Verification items for the finished model (mm, model axes). A direction names the side the tool comes from. Round coordinates to 2 decimals unless told otherwise and drop trailing zeros. Order: outer loops, then holes, each group sorted by start corner. A loop starts at its lowest first (then second) coordinate and runs counter-clockwise, first axis right, second up. Notation, with made-up numbers: (36, 64) -> (87, 64) arc R11 cw to (87, 76) -> close; hole circle Ø9 at (55.5, -25). An arc over 180 degrees is marked (long way). Put each result on its own line as item: value.
```python
from build123d import *

# Parameters (mm, degrees)
BOSS_EXTRUDE1_DEPTH = 15
BOSS_EXTRUDE2_DEPTH = 42
CUT_EXTRUDE1_REACH  = 101.75
SKETCH2_R           = 3.5


with BuildPart() as part:
    # Sketch1 → Boss-Extrude1 (new body)
    with BuildSketch(Plane(origin=(0, 0, 0), x_dir=(1, 0, 0), z_dir=(0, 1, 0))):
        with BuildLine():
            Line((74, 0), (27, 0))
            Line((27, 0), (27, -31))
            Line((27, -31), (62, -31))
            Line((62, -31), (112, -23))
            Line((112, -23), (112, -9))
            Line((112, -9), (83, -9))
            ThreePointArc((83, -9), (76.636038969, -6.363961031), (74, 0))
        make_face()
        with BuildLine():
            Line((27, 31), (27, 0))
            Line((27, 0), (74, 0))
            ThreePointArc((74, 0), (76.636038969, 6.363961031), (83, 9))
            Line((83, 9), (112, 9))
            Line((112, 9), (112, 23))
            Line((112, 23), (62, 31))
            Line((62, 31), (27, 31))
        make_face()
    extrude(amount=BOSS_EXTRUDE1_DEPTH)

    # Sketch1_3 → Boss-Extrude2 (add)
    with BuildSketch(Plane(origin=(0, 0, 0), x_dir=(1, 0, 0), z_dir=(0, 1, 0))):
        Polygon((7, 20), (0, 20), (0, 0), (27, 0), (27, 31), (7, 31), align=None)
        Polygon((27, 0), (0, 0), (0, -20), (7, -20), (7, -31), (27, -31), align=None)
    extrude(amount=BOSS_EXTRUDE2_DEPTH)

    # Sketch2 → Cut-Extrude1 (cut, up to next)
    with BuildSketch(Plane(origin=(27, 0, 0), x_dir=(0, 0, -1), z_dir=(1, 0, 0)), mode=Mode.PRIVATE) as cut_extrude1_sk1:
        with Locations((0, 33)):
            Circle(SKETCH2_R)
    cut_extrude1_tool1 = extrude(cut_extrude1_sk1.sketch, amount=-CUT_EXTRUDE1_REACH, mode=Mode.PRIVATE) & part.part
    # Sketch2 → Cut-Extrude1 (cut, up to next)
    with BuildSketch(Plane(origin=(27, 0, 0), x_dir=(0, 0, -1), z_dir=(1, 0, 0)), mode=Mode.PRIVATE) as cut_extrude1_sk2:
        Polygon((-31, 30), (-8.431282416, 42), (-31, 42), align=None)
    cut_extrude1_tool2 = extrude(cut_extrude1_sk2.sketch, amount=-CUT_EXTRUDE1_REACH, mode=Mode.PRIVATE) & part.part
    # Sketch2 → Cut-Extrude1 (cut, up to next)
    with BuildSketch(Plane(origin=(27, 0, 0), x_dir=(0, 0, -1), z_dir=(1, 0, 0)), mode=Mode.PRIVATE) as cut_extrude1_sk3:
        Polygon((31, 42), (8.431282416, 42), (31, 30), align=None)
    cut_extrude1_tool3 = extrude(cut_extrude1_sk3.sketch, amount=-CUT_EXTRUDE1_REACH, mode=Mode.PRIVATE) & part.part
    add(cut_extrude1_tool1.solids().sort_by_distance((27, 33, 0))[0], mode=Mode.SUBTRACT)
    add(cut_extrude1_tool2.solids().sort_by_distance((27, 38, 23.477094))[0], mode=Mode.SUBTRACT)
    add(cut_extrude1_tool3.solids().sort_by_distance((27, 38, -23.477094))[0], mode=Mode.SUBTRACT)


solid = part.part
```
Item 1: Depth check by flat-ended pin: pin 1 Ø4 at (x, z) = (52, -14) entering from +Y; pin 2 Ø5.5 at (x, y) = (2.5, 12.5) entering from -Z; pin 3 Ø5 at (y, z) = (28, -20.5) entering from +X. Enter the tip coordinate at first touch or a pass-through.
Geometry check:
pin 1: y = 15
pin 2: z = -20
pin 3: x = 27
Item 2: Release check for a two-part mould opening along Z. For faces 6 (the face through (7, 18, -26)), 7 (the face through (97, 7, -9)), 8 (the face through (29, 11, -31)) record: pulls with the +Z half, pulls with the -Z half, needs draft (parallel to the pull), parting line crosses it, or undercut.
Geometry check:
face 6: needs draft
face 7: undercut
face 8: pulls with the -Z half
Item 3: Sectioned sample at C-C, the plane x = 25. Record the boundary of the cut face in (y, z), then the cut area to 3 significant figures.
Geometry check:
outline: (0, -31) -> (30, -31) -> (42, -8.43) -> (42, 8.43) -> (30, 31) -> (0, 31) -> close; hole circle Ø7 at (33, 0)
area: 2,290 mm2
Item 4: Tool access check on faces 1 (the face through (4, 18, -20)), 2 (the face through (87, 7, 27)), 3 (the face through (13.689, 36.084, -19.558)), 4 (the face through (3, 18, 20)), 5 (the face through (59, 15, 0)). Record the directions out of +Z, -Z, +X, -X, +Y, -Y that give a thin tool (end or side, any length) a straight path to the whole face; none if there is none.
Geometry check:
face 1: -Z, -X, +Y, -Y
face 2: +Z, +X, +Y, -Y
face 3: -Z, +X, -X, +Y
face 4: +Z, -X, +Y, -Y
face 5: +Z, -Z, +X, +Y
Item 5: Material ranges on line 1 along Y through (x, z) = (16, 0); line 2 along X through (y, z) = (35.5, -6); line 3 along Y through (x, z) = (53, -3.5), recorded low to high.
Geometry check:
line 1: 0 to 29.5, 36.5 to 42
line 2: 0 to 27
line 3: 0 to 15
Item 6: Sectioned sample at D-D, the plane y = 33. Record the boundary of the cut face in (x, z), then the cut area to 3 significant figures.
Geometry check:
outline: (0, -20) -> (7, -20) -> (7, -25.36) -> (27, -25.36) -> (27, -3.5) -> (0, -3.5) -> close; (0, 3.5) -> (27, 3.5) -> (27, 25.36) -> (7, 25.36) -> (7, 20) -> (0, 20) -> close
area: 1,110 mm2
Item 7: Sectioned sample at A-A, the plane x = 89. Record the boundary of the cut face in (y, z).
Geometry check:
outline: (0, -26.68) -> (15, -26.68) -> (15, -9) -> (0, -9) -> close; (0, 9) -> (15, 9) -> (15, 26.68) -> (0, 26.68) -> close
Item 8: Sectioned sample at B-B, the plane y = 7.5. Record the boundary of the cut face in (x, z).
Geometry check:
outline: (0, -20) -> (7, -20) -> (7, -31) -> (62, -31) -> (112, -23) -> (112, -9) -> (83, -9) arc R9 cw to (83, 9) -> (112, 9) -> (112, 23) -> (62, 31) -> (7, 31) -> (7, 20) -> (0, 20) -> close
